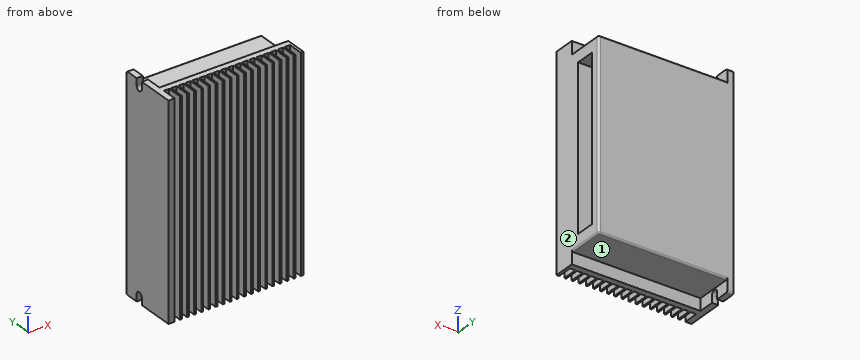
```python
from build123d import *

# Parameters (mm, degrees)
F2_DEPTH = 59.25
F1_W     = 72.5
F1_H     = 21
F3_DEPTH = 52.5
F5_DEPTH = 3.5
F6_W     = 11
F6_H     = 91
F7_DEPTH = 25
F8_R     = 1


with BuildPart() as f2:
    # F1 (on Top) → F2 (new body, symmetric)
    with BuildSketch(Plane.XY):
        Polygon((-34.5, 16.5), (-38, 16.5), (-38, -16.5), (-34.5, -16.5), (-34.5, -8), (-31.5, -8), (-31.5, -16.5), (-30.5, -16.5), (-30.5, -8), (-27.5, -8), (-27.5, -16.5), (-26.5, -16.5), (-26.5, -8), (-23.5, -8), (-23.5, -16.5), (-22.5, -16.5), (-22.5, -8), (-19.5, -8), (-19.5, -16.5), (-18.5, -16.5), (-18.5, -8), (-15.5, -8), (-15.5, -16.5), (-14.5, -16.5), (-14.5, -8), (-11.5, -8), (-11.5, -16.5), (-10.5, -16.5), (-10.5, -8), (-7.5, -8), (-7.5, -16.5), (-6.5, -16.5), (-6.5, -8), (-3.5, -8), (-3.5, -16.5), (-2.5, -16.5), (-2.5, -8), (0.5, -8), (0.5, -16.5), (1.5, -16.5), (1.5, -8), (4.5, -8), (4.5, -16.5), (5.5, -16.5), (5.5, -8), (8.5, -8), (8.5, -16.5), (9.5, -16.5), (9.5, -8), (12.5, -8), (12.5, -16.5), (13.5, -16.5), (13.5, -8), (16.5, -8), (16.5, -16.5), (17.5, -16.5), (17.5, -8), (20.5, -8), (20.5, -16.5), (21.5, -16.5), (21.5, -8), (24.5, -8), (24.5, -16.5), (25.5, -16.5), (25.5, -8), (28.5, -8), (28.5, -16.5), (29.5, -16.5), (29.5, -8), (32.5, -8), (32.5, -16.5), (33.5, -16.5), (33.5, -8), (36.5, -8), (36.5, -16.5), (38, -16.5), (38, -4.5), (-34.5, -4.5), align=None)
    extrude(amount=F2_DEPTH, both=True)

    # F1 (on Top) → F3 (join, symmetric)
    with BuildSketch(Plane.XY):
        with Locations((1.75, 6)):
            Rectangle(F1_W, F1_H)
    extrude(amount=F3_DEPTH, both=True)

    # F4 (on face) → F5 (cut, through all)
    with BuildSketch(Plane(origin=(-38, 0, 0), x_dir=(0, -1, 0), z_dir=(-1, 0, 0))):
        with BuildLine():
            Line((-4.5, 59.25), (-8.5, 59.25))
            Line((-8.5, 59.25), (-8.5, 55.25))
            ThreePointArc((-8.5, 55.25), (-6.5, 53.25), (-4.5, 55.25))
            Line((-4.5, 55.25), (-4.5, 59.25))
        make_face()
        with BuildLine():
            Line((-8.5, -55.25), (-8.5, -59.25))
            Line((-8.5, -59.25), (-4.5, -59.25))
            Line((-4.5, -59.25), (-4.5, -55.25))
            ThreePointArc((-4.5, -55.25), (-6.5, -53.25), (-8.5, -55.25))
        make_face()
    extrude(amount=-F5_DEPTH, mode=Mode.SUBTRACT)

    # F6 (on face) → F7 (cut)
    with BuildSketch(Plane.YZ.offset(38)):
        with Locations((6, 0)):
            Rectangle(F6_W, F6_H)
    extrude(amount=-F7_DEPTH, mode=Mode.SUBTRACT)

    # F8
    f8_edges = [f2.edges().sort_by_distance(p)[0] for p in [
        (38, 6, 52.5),
        (1.75, 16.5, 52.5),
        (38, 16.5, 0),
        (-36.25, 16.5, 59.25),
        (1.75, 16.5, -52.5),
        (38, 6, -52.5),
        (-36.25, 16.5, -59.25),
    ]]
    fillet(f8_edges, radius=F8_R)


solid = f2.part
```
Geometry check sheet. Reference: the model listing, model coordinates, mm. Face numbers are marked on the shaded views. A direction names the side the tool comes from. Round coordinates to 2 decimals unless told otherwise and drop trailing zeros. Loops run counter-clockwise (first coordinate to the right, second up) from the corner with the lowest first, then second, coordinate; pieces in that order, holes last. Notation, with made-up numbers: (40.5, -11.75) -> (72.5, -11.75) arc R16 ccw to (72.5, -1.75) -> close; hole circle Ø7 at (-37.5, 0). An arc over 180 degrees is marked (long way). Use a Markdown table: item, result.
(1) Sectioned sample at C-C (y = -9.5). Give the number of separate pieces and of enclosed holes in the cut face, then the cut area to 3 significant figures.
Calculated:
| item | result |
|---|---|
| separate pieces | 19 |
| enclosed holes | 0 |
| area | 2,610 mm² |
(2) Set-up check for the marked faces 1 and 2: record each of +Z, -Z, +X, -X, +Y, -Y from which the full face is reachable in a straight line by a thin tool's end or side.
Calculated:
| item | result |
|---|---|
| face 1 | -Z, +X, +Y |
| face 2 | +Z, -Z, +X, +Y, -Y |
(3) Go/stop test with flat-tipped pins: P1, Ø0.9, axis at x = -29, z = 18.5, coming from the -Y side; P2, Ø1.5, axis at x = 13.5, y = 2.5, coming from the -Z side; P3, Ø5, axis at x = 17.5, y = 1.5, coming from the +Z side. Record where each tip stops, or that it passes through.
Calculated:
| item | result |
|---|---|
| P1 | y = -8 |
| P2 | z = -52.5 |
| P3 | z = 52.5 |
(4) Sectioned sample at A-A (x = 19). Enter the section's corners in (y, z).
Calculated:
| item | result |
|---|---|
| outline | (-8, -59.25) -> (-4.5, -59.25) -> (-4.5, -52.5) -> (15.5, -52.5) arc R1 ccw to (16.5, -51.5) -> (16.5, 51.5) arc R1 ccw to (15.5, 52.5) -> (-4.5, 52.5) -> (-4.5, 59.25) -> (-8, 59.25) -> close; hole (0.5, -45.5) -> (11.5, -45.5) -> (11.5, 45.5) -> (0.5, 45.5) -> close |
(5) Sectioned sample at B-B (y = 6.5). Enter the section's corners in (x, z).
Calculated:
| item | result |
|---|---|
| outline | (-38, -53.25) -> (-34.5, -53.25) -> (-34.5, -52.5) -> (37, -52.5) arc R1 ccw to (38, -51.5) -> (38, -45.5) -> (13, -45.5) -> (13, 45.5) -> (38, 45.5) -> (38, 51.5) arc R1 ccw to (37, 52.5) -> (-34.5, 52.5) -> (-34.5, 53.25) -> (-38, 53.25) -> close |
(6) Scan lines: probe 1 along Y at (x, z) = (20, 41); probe 2 along Z at (x, y) = (31, 3); probe 3 along Y at (x, z) = (-1, 38). Record each from-to range of solid material in increasing order.
Calculated:
| item | result |
|---|---|
| probe 1 | -8 to 0.5, 11.5 to 16.5 |
| probe 2 | -52.5 to -45.5, 45.5 to 52.5 |
| probe 3 | -8 to 16.5 |
